```python
from build123d import *

# Parameters (mm, degrees)
SKETCH3_R          = 3.275
CUT_EXTRUDE1_DEPTH = 27.529839572
CHAMFER1_SIZE      = 0.3


with BuildPart() as part:
    # Sketch2 → Revolve1 (revolve)
    with BuildSketch(Plane.XY, mode=Mode.PRIVATE) as revolve1_sk:
        with BuildLine():
            Line((0, 0), (0, 4.7625))
            Line((0, 4.7625), (18.4546875, 4.7625))
            Line((18.4546875, 4.7625), (18.4546875, 1.5875))
            Line((18.4546875, 1.5875), (15.2796875, 1.5875))
            ThreePointArc((15.2796875, 1.5875), (14.940933498, 1.727816502), (15.08125, 1.3890625))
            Line((15.08125, 1.3890625), (15.08125, 0))
            Line((15.08125, 0), (0, 0))
        make_face()
    revolve(revolve1_sk.sketch.rotate(Axis((0, 0, 0), (0, 1, 0)), 90), axis=Axis((0, 0, 0), (0, 1, 0)))

    # Sketch3 → Cut-Extrude1 (cut, through all)
    with BuildSketch(Plane(origin=(0, 0, 0), x_dir=(-1, 0, 0), z_dir=(0, -1, 0))):
        with Locations(Location((0, 0, 0), (0, 0, 90))):
            Circle(SKETCH3_R)
    extrude(amount=-CUT_EXTRUDE1_DEPTH, mode=Mode.SUBTRACT)

    # Chamfer1
    chamfer1_edges = [part.edges().sort_by_distance(p)[0] for p in [
        (0, 4.7625, 3.275),
        (0, 0, 3.275),
        (0, 4.7625, 18.4546875),
        (0, 0, 15.08125),
    ]]
    chamfer(chamfer1_edges, length=CHAMFER1_SIZE)


solid = part.part
```
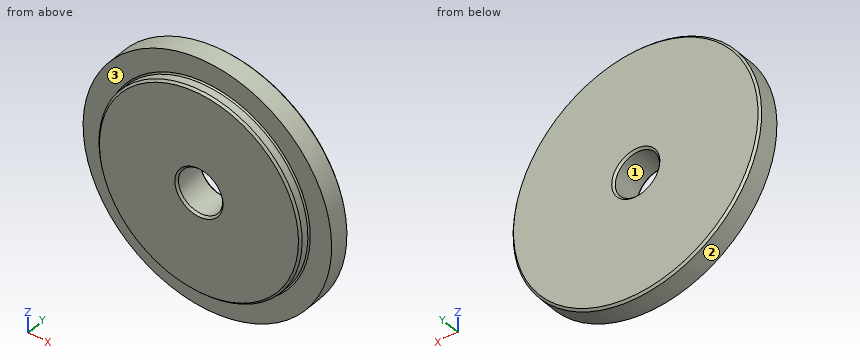
Geometry check sheet. Reference: the model listing, model coordinates, mm. Face numbers are marked on the shaded views. Round coordinates to 2 decimals unless told otherwise and drop trailing zeros. Loops run counter-clockwise (first coordinate to the right, second up) from the corner with the lowest first, then second, coordinate; pieces in that order, holes last. Notation, with made-up numbers: (87.5, -33.75) - (100.5, -33.75) arc R7 cw to (100.5, -22.75) - close; hole circle Ø6 at (52.5, 56). An arc over 180 degrees is marked (long way). Write each question's results on one line, items separated by ' | '. Start each with the question number.
Q1. Gauge pin test, flat end, axial feed: P1, Ø1, axis at y = 2.5, z = 13.5, coming from the -X side. Record the tip position at first contact, or that the pin passes through.
Q2. Cross-section at C-C on y = 2.35. Enter the section's corners in (x, z) (3 decimals), and give its area (3 significant figures).
Q3. Thickness scan on line 1 (X direction, y = 2.8, z = 0) (3 decimals); line 2 (X direction, y = 1.3, z = 0) (3 decimals); line 3 (Y direction, x = 16, z = 5.5). Record the ranges inside material, lowest first. Write a range as [from, to].
Q4. Release check for a two-part mould opening along Z. For the marked faces 1, 2 and 3 record: +Z half, -Z half, draft (parallel to the pull), parting line (faces both ways), or undercut.
Answers below:
1) P1: stops at x = -13.1
2) outline: circle Ø36.909 at (0, 0); hole circle Ø6.55 at (0, 0) | area: 1,040 mm²
3) line 1: x = [-18.455, -3.275], [3.275, 18.455] | line 2: x = [-15.081, -3.275], [3.275, 15.081] | line 3: y = [1.59, 4.76]
4) face 1: undercut | face 2: parting line | face 3: draft
